For this review, take the finished solid that the model builds, in its own axes (mm). A direction names the side the tool comes from. Coordinates: 2 decimals unless noted, no trailing zeros. Order: outer loops, then holes, each group sorted by start corner. A loop starts at its lowest first (then second) coordinate and runs counter-clockwise, first axis right, second up. Notation, with made-up numbers: M 81.5,-33.75 L 123.5,-33.75 A28 ccw 123.5,-2.75 Z; hole C 14,-6 d1. An arc over 180 degrees is marked long. Use CSV: the item, a comma, the result in double quotes.
Autodesk Inventor part; units mm, degrees
ref_plane "YZ Plane" through (0, 0, 0) normal (1, 0, 0) x (0, 1, 0)
ref_plane "XZ Plane" through (0, 0, 0) normal (0, 1, 0) x (-1, 0, 0)
ref_plane "XY Plane" through (0, 0, 0) normal (0, 0, 1) x (1, 0, 0)
sketch "Sketch1" plane through (0, 0, 0) normal (0, 1, 0) x (-1, 0, 0)
  line L0 (0, 0) -> (-27, 0)
  line L1 (-27, 0) -> (-27, -26.6)
  line L2 (-27, -26.6) -> (0, -26.6)
  line L3 (0, -26.6) -> (0, 0)
  dimension "d0" = 27
  dimension "d1" = 26.6
extrude "Extrusion1" add sketch "Sketch1" along normal blind 3
sketch "Sketch2" plane through (0, 3, 0) normal (0, 1, 0) x (1, 0, 0)
  line L0 (0, 26.6) -> (0, 0)
  circle A0 centre (0, 13.3) radius 1
  dimension "d4" = 2
extrude "Extrusion2" cut sketch "Sketch2" against normal blind 1
sketch "Sketch3" plane through (0, 3, 0) normal (0, 1, 0) x (1, 0, 0)
  point P0 (0, 0)
  point P1 (3.4, 3.2)
  point P2 (23.6, 3.2)
  point P3 (23.6, 23.4)
  point P4 (3.4, 23.4)
hole "Hole1" at (3.4, 3, -3.2) at (23.6, 3, -3.2) at (23.6, 3, -23.4) at (3.4, 3, -23.4) direction (0, -1, 0) diameter 2 end through all
sketch "Sketch4" plane through (0, 3, 0) normal (0, 1, 0) x (1, 0, 0)
  point P0 (0, 0)
properties part number "Top mount"
Item 1: For faces 4 (the face through (0.4, 2, -13.3)), 5 (the face through (3.4, 1.5, -24.4)), list the 3-axis set-ups (+Z, -Z, +X, -X, +Y, -Y) from which the entire face can be reached by the end or side of a thin tool; tool diameter is ignored.
Solutions:
face 4,"-X, +Y"
face 5,"+Y, -Y"
Item 2: Add section B-B on y = 1.5. State the section outline as (x, z) points, and give its area (3 significant figures).
Solutions:
outline,"M 0,-26.6 L 27,-26.6 L 27,0 L 0,0 Z; hole C 3.4,-23.4 d2; hole C 3.4,-3.2 d2; hole C 23.6,-23.4 d2; hole C 23.6,-3.2 d2"
area,"706 mm^2"
Item 3: Clearance check with a flat-ended pin moving along its axis: pin 1 Ø1.2 at (x, z) = (3.4, -23.4) entering from -Y. State where the tip first meets the part, or that it passes through.
Solutions:
pin 1,"through"
Item 4: Draft analysis for pull direction Z (two halves, no side actions). For faces 1 (the face through (0, 1, -13)), 2 (the face through (4.29, 1.48, -2.74)), 3 (the face through (13, 1, 0)), state which applies: released by +Z, released by -Z, zero draft, split by the parting line, or undercut.
Solutions:
face 1,"zero draft"
face 2,"undercut"
face 3,"released by +Z"
Item 5: Add section A-A on x = 23.6. State the section outline as (y, z) points, and give its area (3 significant figures).
Solutions:
outline,"M 0,-26.6 L 3,-26.6 L 3,-24.4 L 0,-24.4 Z; M 0,-22.4 L 3,-22.4 L 3,-4.2 L 0,-4.2 Z; M 0,-2.2 L 3,-2.2 L 3,0 L 0,0 Z"
area,"67.8 mm^2"
Item 6: To check wall thickness, follow line 1 along Z through (x, y) = (23.6, 2.3); line 2 along X through (y, z) = (1.4, -23.4); line 3 along Z through (x, y) = (4.25, 0.55). State the ranges of each line that lie inside material, in increasing order. Write a range as [from, to].
Solutions:
line 1,"[-26.6, -24.4], [-22.4, -4.2], [-2.2, 0]"
line 2,"[0, 2.4], [4.4, 22.6], [24.6, 27]"
line 3,"[-26.6, -23.93], [-22.87, -3.73], [-2.67, 0]"
Item 7: Add section C-C on z = -23.4. State the section outline as (x, y) points.
Solutions:
outline,"M 0,0 L 2.4,0 L 2.4,3 L 0,3 Z; M 4.4,0 L 22.6,0 L 22.6,3 L 4.4,3 Z; M 24.6,0 L 27,0 L 27,3 L 24.6,3 Z"
